Could you check a few things on this drawing? It's one solid part, dimensions in mm from its lowest x, y, z. Coordinates: 2 decimals unless noted, no trailing zeros. Order: outer loops, then holes, each group sorted by start corner. A loop starts at its lowest first (then second) coordinate and runs counter-clockwise, first axis right, second up.
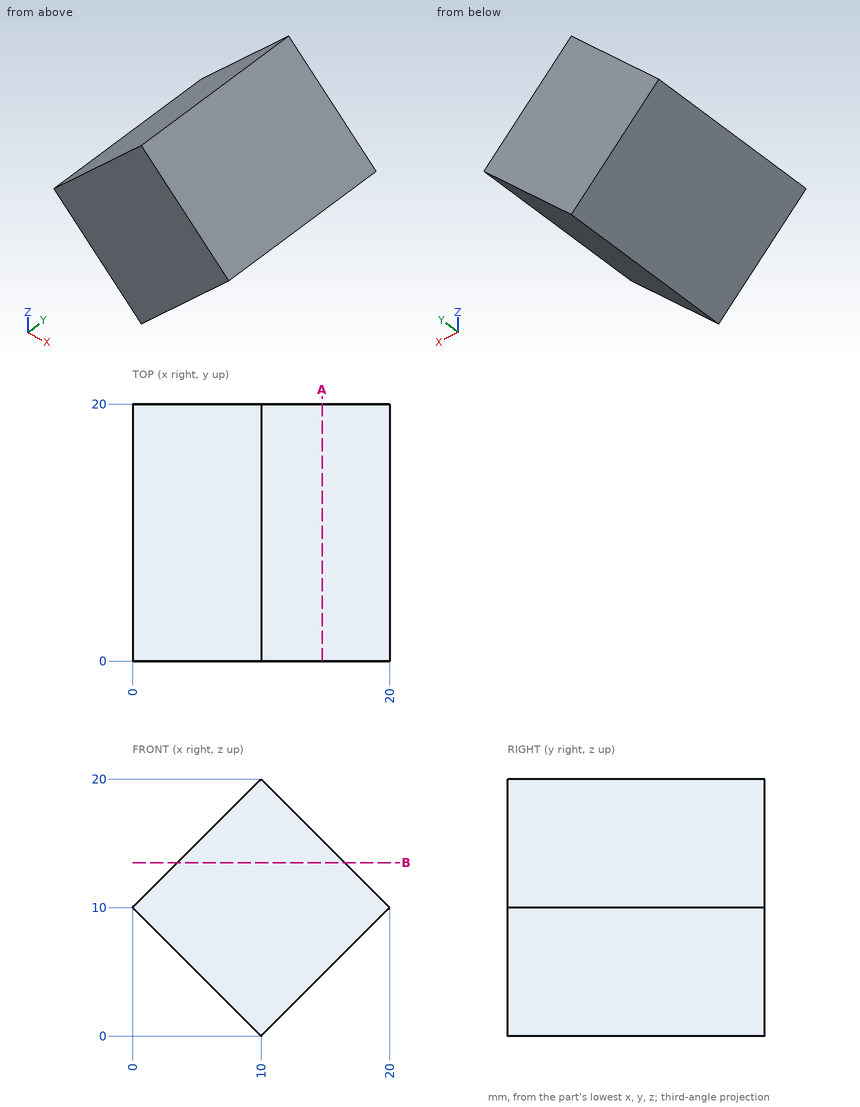
1. I'm going to push flat-ended pins straight in: pin 1 (8 mm diameter, centred on x = 13.5, z = 12, fed in from -Y); pin 2 (4 mm diameter, centred on y = 6.5, z = 15.5, fed in from +X); pin 3 (10 mm diameter, centred on y = 9, z = 3.5, fed in from -X); pin 4 (1 mm diameter, centred on y = 12.5, z = 9, fed in from -X). Where does each tip first touch, or does it pass through?
Completed:
pin 1: stops at y = 0
pin 2: stops at x = 16.5
pin 3: stops at x = 1.5
pin 4: stops at x = 0.5
2. Imagine slicing it at B-B on z = 13.5. Please give me the cut outline in (x, y).
Completed:
outline: (3.5, 0) - (16.5, 0) - (16.5, 20) - (3.5, 20) - close
3. Please list where these lines run through material, in increasing order: probe 1 along X at (y, z) = (19, 1.75); probe 2 along Z at (x, y) = (7, 18.75); probe 3 along X at (y, z) = (10.75, 15.25).
Completed:
probe 1: x = 8.25 to 11.75
probe 2: z = 3 to 17
probe 3: x = 5.25 to 14.75
4. Imagine slicing it at A-A on x = 14.75. Please give me the cut outline in (y, z).
Completed:
outline: (0, 4.75) - (20, 4.75) - (20, 15.25) - (0, 15.25) - close
